Could you check a few things on this model? Use its own coordinates, in mm. A direction names the side the tool comes from. Give positions to 0.01 mm unless a question says otherwise; leave off trailing zeros. Write each loop counter-clockwise with the first axis right and the second up, starting at its lowest first coordinate (ties: lowest second). Pieces come first, ordered by that corner, then holes. Notation, with made-up numbers: M 77,-38.5 L 127,-38.5 A19 cw 127,-15.5 Z; hole C 73,52 d11. An arc over 180 degrees is marked long. Use one line per item in the form item = value.
from build123d import *
from OCP.BRepFilletAPI import BRepFilletAPI_MakeChamfer

# Parameters (mm, degrees)
SKETCH1_W              = 16
SKETCH1_H              = 17.3
BOSS_EXTRUDE1_DEPTH    = 6.5
SKETCH2_W              = 4
SKETCH2_H              = 3.85
BOSS_EXTRUDE2_DEPTH    = 2
BOSS_EXTRUDE3_DEPTH    = 2
SKETCH4_R              = 4.5
BOSS_EXTRUDE4_DEPTH    = 5
SKETCH5_R              = 3.5
BOSS_EXTRUDE5_DEPTH    = 3
BOSS_EXTRUDE6_DEPTH    = 7
CHAMFER1_SIZE          = 1.5
CHAMFER1_SIZE2         = 0.866025404
SKETCH7_W              = 0.75
SKETCH7_H              = 1.85
BOSS_EXTRUDE7_DEPTH    = 1
SKETCH8_W              = 0.75
SKETCH8_H              = 0.75
BOSS_EXTRUDE8_DEPTH    = 3.7
FILLET1_R              = 0.4
LPATTERN1_COUNT        = 2
LPATTERN1_PITCH        = 5
FILLET1_OF_LPATTERN1_R = 0.4
MIRROR1_START          = 4.625
MIRROR1_DEPTH          = 0.75
SKETCH10_W             = 0.4
SKETCH10_H             = 2
BOSS_EXTRUDE9_DEPTH    = 5.5
FILLET2_R              = 0.4
FILLET3_R              = 1
FILLET2_OF_MIRROR2_R   = 0.4
FILLET3_OF_MIRROR2_R   = 1


# Read off the part's stored shape, not the designer's step: Mirror1
with BuildPart() as part:
    # Sketch1 → Boss-Extrude1 (new body)
    with BuildSketch(Plane.XY):
        Rectangle(SKETCH1_W, SKETCH1_H)
    extrude(amount=BOSS_EXTRUDE1_DEPTH)

    # Sketch2 → Boss-Extrude2 (add)
    with BuildSketch(Plane.XY.offset(6.5)):
        with Locations((0, -10.575)):
            Rectangle(SKETCH2_W, SKETCH2_H)
    extrude(amount=-BOSS_EXTRUDE2_DEPTH)

    # Sketch3 → Boss-Extrude3 (add)
    with BuildSketch(Plane.XY.offset(6.5)):
        with BuildLine():
            Line((-1.299038106, -8.55), (1.299038106, -8.55))
            ThreePointArc((1.299038106, -8.55), (0, -10.8), (-1.299038106, -8.55))
        make_face()
    extrude(amount=BOSS_EXTRUDE3_DEPTH)

    # Sketch4 → Boss-Extrude4 (add)
    with BuildSketch(Plane.XY.offset(6.5)):
        with Locations(Location((0, 0, 0), (0, 0, 180))):
            Circle(SKETCH4_R)
    extrude(amount=BOSS_EXTRUDE4_DEPTH)

    # Sketch5 → Boss-Extrude5 (add)
    with BuildSketch(Plane.XY.offset(11.5)):
        Circle(SKETCH5_R)
    extrude(amount=BOSS_EXTRUDE5_DEPTH)

    # Sketch6 → Boss-Extrude6 (add)
    with BuildSketch(Plane.XY.offset(14.5)):
        with BuildLine():
            Line((-3.354101966, 1), (3.354101966, 1))
            ThreePointArc((3.354101966, 1), (0, -3.5), (-3.354101966, 1))
        make_face()
    extrude(amount=BOSS_EXTRUDE6_DEPTH)

    # Chamfer1: one chamfer whose edges measure the first distance from different faces: ONE call of the kernel's chamfer builder (chamfer() names one face for all edges)
    chamfer1_edges_1 = [part.edges().sort_by_distance(p)[0] for p in [
        (0, -3.5, 21.5),
    ]]
    chamfer1_side_1 = [part.faces().sort_by_distance(p)[0] for p in [
        (0, -3.5, 18),
    ]]
    chamfer1_edges_2 = [part.edges().sort_by_distance(p)[0] for p in [
        (0, 1, 21.5),
    ]]
    chamfer1_side_2 = [part.faces().sort_by_distance(p)[0] for p in [
        (0, 1, 18),
    ]]
    chamfer1 = BRepFilletAPI_MakeChamfer(part.part.solid().wrapped)
    for e in chamfer1_edges_1:
        chamfer1.Add(CHAMFER1_SIZE, CHAMFER1_SIZE2, e.wrapped, chamfer1_side_1[0].wrapped)  # the first distance lies on this face
    for e in chamfer1_edges_2:
        chamfer1.Add(CHAMFER1_SIZE, CHAMFER1_SIZE2, e.wrapped, chamfer1_side_2[0].wrapped)  # the first distance lies on this face
    add(Compound.cast(chamfer1.Shape()), mode=Mode.REPLACE)

    # Sketch7 → Boss-Extrude7 (add)
    with BuildSketch(Plane(origin=(0, 0, 2), x_dir=(-1, 0, 0), z_dir=(0, 0, -1))):
        with Locations((0, -9.575)):
            Rectangle(SKETCH7_W, SKETCH7_H)
    boss_extrude7 = extrude(amount=BOSS_EXTRUDE7_DEPTH)

    # Sketch8 → Boss-Extrude8 (add)
    with BuildSketch(Plane(origin=(0, 0, 1), x_dir=(-1, 0, 0), z_dir=(0, 0, -1))):
        with Locations((0, -10.125)):
            Rectangle(SKETCH8_W, SKETCH8_H)
    boss_extrude8 = extrude(amount=BOSS_EXTRUDE8_DEPTH)

    # Fillet1
    fillet1_edges = [part.edges().sort_by_distance(p)[0] for p in [
        (0, -10.5, 2),
        (0, -9.75, 1),
    ]]
    fillet(fillet1_edges, radius=FILLET1_R)

    # LPattern1: Boss-Extrude7, Boss-Extrude8 ×2
    with Locations(*[(-i * LPATTERN1_PITCH, 0, 0) for i in range(1, LPATTERN1_COUNT)]):
        add(boss_extrude7)
        add(boss_extrude8)

    # Fillet1 of LPattern1
    fillet1_of_lpattern1_edges = [part.edges().sort_by_distance(p)[0] for p in [
        (-5, -10.5, 2),
        (-5, -9.75, 1),
    ]]
    fillet(fillet1_of_lpattern1_edges, radius=FILLET1_OF_LPATTERN1_R)

    # Mirror1 outline → Mirror1 (add)
    with BuildSketch(Plane.YZ.offset(MIRROR1_START)):
        with BuildLine():
            ThreePointArc((-9.75, 0.6), (-9.632842712, 0.882842712), (-9.35, 1))
            Line((-9.35, 1), (-8.65, 1))
            Line((-8.65, 1), (-8.65, 2))
            Line((-8.65, 2), (-10.1, 2))
            ThreePointArc((-10.1, 2), (-10.382842712, 1.882842712), (-10.5, 1.6))
            Line((-10.5, 1.6), (-10.5, -2.7))
            Line((-10.5, -2.7), (-9.75, -2.7))
            Line((-9.75, -2.7), (-9.75, 0.6))
        make_face()
    extrude(amount=MIRROR1_DEPTH)

    # Sketch10 → Boss-Extrude9 (add)
    with BuildSketch(Plane(origin=(0, 0, 2), x_dir=(-1, 0, 0), z_dir=(0, 0, -1))):
        with Locations((8.2, 0)):
            Rectangle(SKETCH10_W, SKETCH10_H)
    boss_extrude9 = extrude(amount=BOSS_EXTRUDE9_DEPTH)

    # Fillet2
    fillet2_edges = [part.edges().sort_by_distance(p)[0] for p in [
        (-8.4, 0, 2),
    ]]
    fillet(fillet2_edges, radius=FILLET2_R - 0.0001)  # a hair under: the kernel refuses the full size

    # Fillet3
    fillet3_edges = [part.edges().sort_by_distance(p)[0] for p in [
        (-8.2, 1, -3.5),
        (-8.2, -1, -3.5),
    ]]
    fillet(fillet3_edges, radius=FILLET3_R - 0.0001)  # a hair under: the kernel refuses the full size

    # Mirror2: Boss-Extrude9 across plane
    add(boss_extrude9.mirror(Plane.ZY))

    # Fillet2 of Mirror2
    fillet2_of_mirror2_edges = [part.edges().sort_by_distance(p)[0] for p in [
        (8.4, 0, 2),
    ]]
    fillet(fillet2_of_mirror2_edges, radius=FILLET2_OF_MIRROR2_R - 0.0001)  # a hair under: the kernel refuses the full size

    # Fillet3 of Mirror2
    fillet3_of_mirror2_edges = [part.edges().sort_by_distance(p)[0] for p in [
        (8.2, 1, -3.5),
        (8.2, -1, -3.5),
    ]]
    fillet(fillet3_of_mirror2_edges, radius=FILLET3_OF_MIRROR2_R - 0.0001)  # a hair under: the kernel refuses the full size


solid = part.part
1) For faces 4 (the flat face through (8, 0, -2)), 5 (the flat face through (0, 1, 17)), 6 (the flat face through (0, -9, 8.5)), 7 (the cylindrical face through (3.32, -3.04, 8.96)), 8 (the flat face through (0, -8.55, 7)), which set-ups out of +Z, -Z, +X, -X, +Y, -Y let a thin tool reach every point of the face, with its end or its side?
Checked values:
face_4 = -Z, +Y, -Y
face_5 = +Z, +X, -X, +Y
face_6 = +Z, +X, -X, -Y
face_7 = +Z
face_8 = +Z, +X, -X
2) Thinking about a two-plate mould opening in Y: for faces 1 (the cylindrical face through (-8.203, -0.699, -3.215)), 2 (the flat face through (0, -11, 4.5)), 3 (the cylindrical face through (0, -10.8, 7.5)), which applies, released by +Y, released by -Y, zero draft, split by the parting line, or undercut?
Checked values:
face_1 = released by -Y
face_2 = zero draft
face_3 = undercut
3) If I drill on L1, parallel to Z at x = 0.5, y = -8.25; L2, parallel to X at y = -2, z = 2.5; L3, parallel to Y at x = 0, z = -0.5, over which ranges is the centre line in solid material (lowest first)?
Checked values:
L1 = 0 to 6.5
L2 = -8 to 8
L3 = -10.5 to -9.75
4) I want a section at B-B, the plane y = -9. Please give me the cut outline in (x, z) (3 decimals).
Checked values:
outline = M -5.375,1 L -4.625,1 L -4.625,2 L -5.375,2 Z; M -2,4.5 L 2,4.5 L 2,6.5 L 1.47,6.5 L 1.47,8.5 L -1.47,8.5 L -1.47,6.5 L -2,6.5 Z; M -0.375,1 L 0.375,1 L 0.375,2 L -0.375,2 Z; M 4.625,1 L 5.375,1 L 5.375,2 L 4.625,2 Z
5) I want a section at D-D, the plane y = -5.75. Please give me the cut outline in (x, z), plus the area to 3 significant figures.
Checked values:
outline = M -8,0 L 8,0 L 8,6.5 L -8,6.5 Z
area = 104 mm2
6) I want a section at C-C, the plane z = 13.5. Please give me the cut outline in (x, y), plus the area to 3 significant figures.
Checked values:
outline = C 0,0 d7
area = 38.5 mm2
7) For pin 1 Ø0.8 at (x, y) = (-5, -10) entering from -Z; pin 2 Ø2 at (y, z) = (-9, -0.5) entering from +X; pin 3 Ø1.5 at (y, z) = (2, 11.5) entering from +X, each with a flat end and sliding along its axis, tell me the tip position at first contact or that it passes through.
Checked values:
pin_1 = -2.7
pin_2 = 8
pin_3 = 4.32
